Source: CAD feature listing. Evaluate the final solid. Frame: model axes, mm. Coordinates: 2 decimals unless noted, no trailing zeros. Write each loop counter-clockwise with the first axis right and the second up, starting at its lowest first coordinate (ties: lowest second). Pieces come first, ordered by that corner, then holes. Notation, with made-up numbers: M 29,-25 L 65,-25 A21 cw 65,2 Z; hole C 70.5,-19 d2. An arc over 180 degrees is marked long. Write item = value, one per line. Start each with the question number.
1. Line query: line 1 along X through (y, z) = (-11, 1.5); line 2 along X through (y, z) = (-20.5, 3.25); line 3 along Y through (x, z) = (-18.5, 6.5). Output: solid intervals per line, ascending.
2. Pin query (flat end, axial travel): pin 1 Ø4 at (y, z) = (29.5, 2.5) entering from +X. Return the tip coordinate at first contact, or that it passes through.
3. Section query A-A (x = -86.5). Output: boundary loops of the cut face in (y, z), then the cut area to 3 significant figures.
4. Section query B-B (x = -49). Output: boundary loops of the cut face in (y, z), then the cut area to 3 significant figures.
```python
from build123d import *

# Parameters (mm, degrees)
EXTRUDE_1_DEPTH     = 10
CUT_EXTRUDE_1_DEPTH = 149.427210809


with BuildPart() as part:
    # Эскиз1_fr → Бобышка-Вытянуть1 (new body)
    with BuildSketch(Plane.XY):
        with BuildLine():
            Line((0, 0), (0, 20))
            add(Edge.make_bspline(
                [(0, 20), (0, 38.146025899), (-14.209474182, 48.611098897), (-41.986949672, 54.649680525)],
                knots=[0, 0, 0, 0, 1, 1, 1, 1], degree=3))
            Line((-41.986949672, 54.649680525), (-103.301225383, 67.978870897))
            add(Edge.make_bspline(
                [(-103.301225383, 67.978870897), (-115.500001367, 70.63077872), (-131.292525164, 63.393306184), (-131.292525164, 43.097715536)],
                knots=[0, 0, 0, 0, 1, 1, 1, 1], degree=3))
            Line((-131.292525164, 43.097715536), (-131.292525164, 0))
            add(Edge.make_bspline(
                [(-97.969549234, -25.769768053), (-112.011160689, -25.769768053), (-131.292525164, -19.025155818), (-131.292525164, 0)],
                knots=[0, 0, 0, 0, 1, 1, 1, 1], degree=3))
            Line((-97.969549234, -25.769768053), (-33.545129103, -25.769768053))
            add(Edge.make_bspline(
                [(-33.545129103, -25.769768053), (-19.444866568, -25.769768053), (0, -19.063757455), (0, 0)],
                knots=[0, 0, 0, 0, 1, 1, 1, 1], degree=3))
        make_face()
    extrude(amount=EXTRUDE_1_DEPTH)

    # Эскиз2_fr → Вырез-Вытянуть1 (cut, through all)
    with BuildSketch(Plane(origin=(0, 0, 0), x_dir=(-1, 0, 0), z_dir=(0, 0, -1))):
        with BuildLine():
            Line((102.429251955, 61.832882372), (104.527789693, 52.179608775))
            ThreePointArc((104.527789693, 52.179608775), (103.259303337, 50.206407776), (101.286102339, 51.474894133))
            Line((101.286102339, 51.474894133), (99.1875646, 61.128167729))
            ThreePointArc((99.1875646, 61.128167729), (100.456050956, 63.101368728), (102.429251955, 61.832882372))
        make_face()
    extrude(amount=-CUT_EXTRUDE_1_DEPTH, mode=Mode.SUBTRACT)


solid = part.part
```
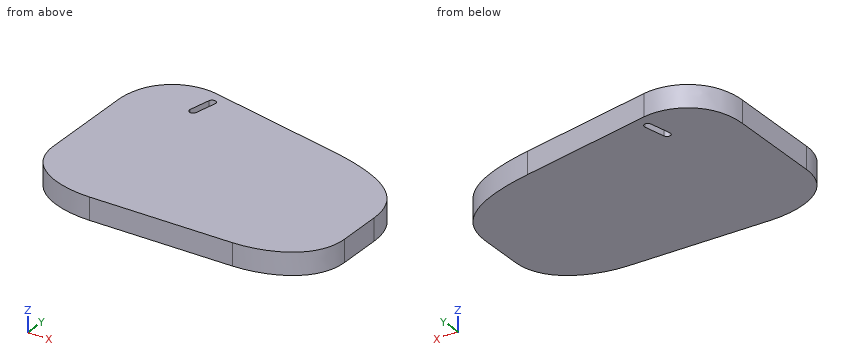
Results are:
q1.line_1 = -128.66 to -2.64
q1.line_2 = -119.09 to -12.27
q1.line_3 = -23.3 to 46.89
q2.pin_1 = -0.92
q3.outline = M -25.77,0 L 64.33,0 L 64.33,10 L -25.77,10 Z
q3.area = 901 mm^2
q4.outline = M -25.77,0 L 56.17,0 L 56.17,10 L -25.77,10 Z
q4.area = 819 mm^2
